```python
from build123d import *

# Parameters (mm, degrees)
SKETCH1_R           = 4.825
BOSS_EXTRUDE1_DEPTH = 85
CHAMFER1_SIZE       = 0.5
CHAMFER2_SIZE       = 0.5
SKETCH2_W           = 0.5
SKETCH2_H           = 0.98


with BuildPart() as part:
    # Sketch1 → Boss-Extrude1 (new body)
    with BuildSketch(Plane.XY):
        Circle(SKETCH1_R)
    extrude(amount=BOSS_EXTRUDE1_DEPTH)

    # Chamfer1
    chamfer1_edges = [part.edges().sort_by_distance(p)[0] for p in [
        (-4.825, 0, 85),
    ]]
    chamfer(chamfer1_edges, length=CHAMFER1_SIZE)

    # Chamfer2
    chamfer2_edges = [part.edges().sort_by_distance(p)[0] for p in [
        (-4.825, 0, 0),
    ]]
    chamfer(chamfer2_edges, length=CHAMFER2_SIZE)

    # Sketch2 → Cut-Revolve1 (revolve, cut)
    with BuildSketch(Plane(origin=(0, 0, 0), x_dir=(1, 0, 0), z_dir=(0, 1, 0)), mode=Mode.PRIVATE) as cut_revolve1_sk:
        with Locations((-4.575, -83.32)):
            Rectangle(SKETCH2_W, SKETCH2_H)
    revolve(cut_revolve1_sk.sketch.rotate(Axis((0, 0, 85), (0, 0, -1)), 180), axis=Axis((0, 0, 85), (0, 0, -1)), mode=Mode.SUBTRACT)


solid = part.part
```
For this review, take the finished solid that the model builds, in its own axes (mm). Round coordinates to 2 decimals unless told otherwise and drop trailing zeros. Write each loop counter-clockwise with the first axis right and the second up, starting at its lowest first coordinate (ties: lowest second). Pieces come first, ordered by that corner, then holes. Notation, with made-up numbers: (-31, 18) -> (-9, 18) arc R29 ccw to (-9, 44) -> close; hole circle Ø11 at (-12, 4). An arc over 180 degrees is marked (long way). Use one line per item in the form item = value.
Q1. The part is to be moulded in two halves that separate along Z. For faces 1 (the flat face through (0, 0, 0)), 2 (the cylindrical face through (4.6, 1.45, 41.09)), 3 (the flat face through (0, 0, 85)), 4 (the cylindrical face through (4.125, -1.299, 83.313)), say which applies: released by +Z, released by -Z, zero draft, split by the parting line, or undercut.
Resolved:
face_1 = released by -Z
face_2 = zero draft
face_3 = released by +Z
face_4 = undercut
Q2. Consider section A-A (z = 36.5). State the section outline as (x, y) points (3 decimals).
Resolved:
outline = circle Ø9.65 at (0, 0)
Q3. Clearance check with flat-ended pins moving along their axes: pin 1 Ø5 at (x, z) = (3.5, 11) entering from +Y; pin 2 Ø1.5 at (x, z) = (-3.5, 44) entering from -Y; pin 3 Ø1 at (y, z) = (2.5, 27) entering from +X. State where each tip first meets the part, or that it passes through.
Resolved:
pin_1 = 4.72
pin_2 = -3.96
pin_3 = 4.39
Q4. To check wall thickness, follow probe 1 along Z at (x, y) = (1.5, -4.5); probe 2 along Z at (x, y) = (-3.25, 3.25); probe 3 along Y at (x, z) = (1.25, 50). State the ranges of each line that lie inside material, in increasing order. Write a range as from..to.
Resolved:
probe_1 = 0.42..82.83, 83.81..84.58
probe_2 = 0.27..82.83, 83.81..84.73
probe_3 = -4.66..4.66
